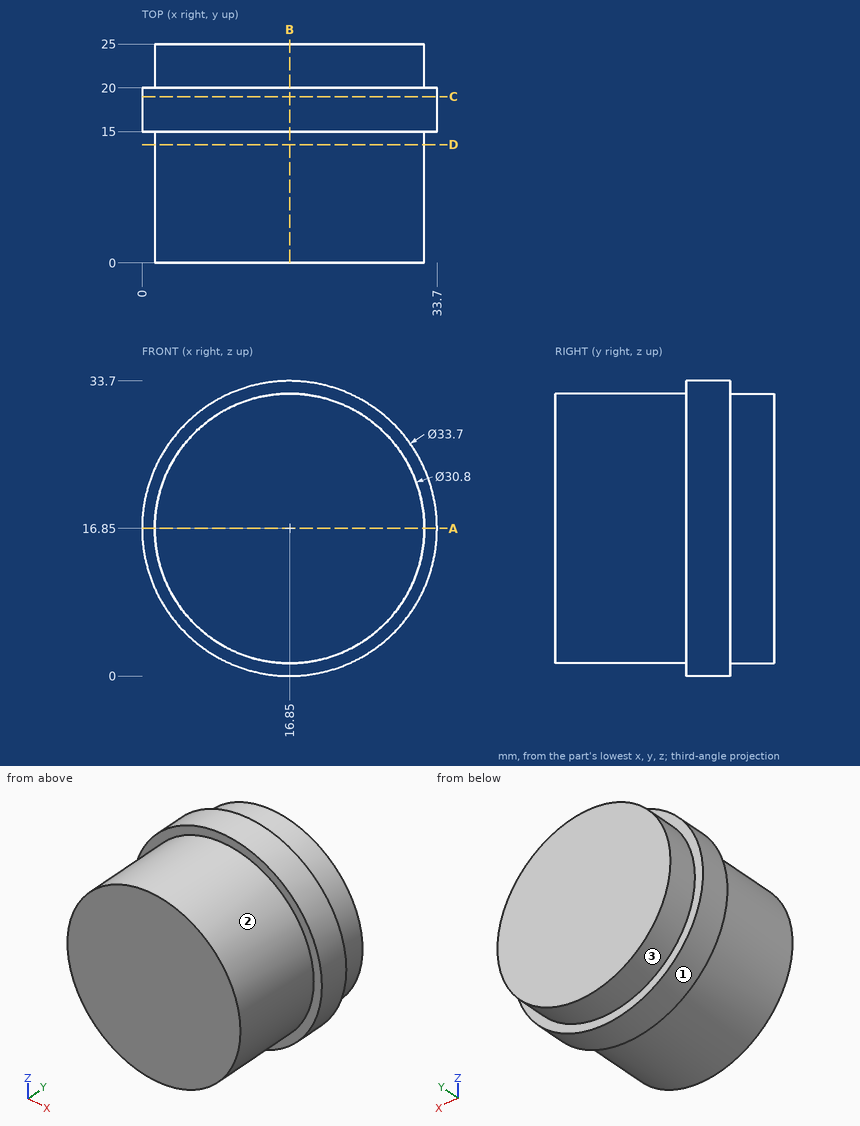
Drawing for the job (mm, zero at the part's lowest x, y, z). A direction names the side the tool comes from. Round coordinates to 2 decimals unless told otherwise and drop trailing zeros. Loops run counter-clockwise (first coordinate to the right, second up) from the corner with the lowest first, then second, coordinate; pieces in that order, holes last. Notation, with made-up numbers: (9.25, -13) - (39.25, -13) arc R12 cw to (39.25, 5) - close; hole circle Ø9 at (40, -9.5). An arc over 180 degrees is marked (long way). Return JSON: item names as keys, results as strings. Group by question number.
Q1. Flat gauge pins, fed straight in: pin 1 Ø1.5 at (y, z) = (14, 3.5) entering from -X; pin 2 Ø12 at (x, y) = (22, 15.5) entering from -Z; pin 3 Ø8 at (y, z) = (7.5, 10.5) entering from -X; pin 4 Ø8 at (y, z) = (16, 7) entering from +X. Where does each tip first touch, or does it go through?
Q2. Band-saw the part on A-A on z = 16.85. Give the cut face in (x, y), plus the area to 4 significant figures.
Q3. Drill centre lines: line 1 along Y through (x, z) = (8, 30); line 2 along Z through (x, y) = (16, 23.5); line 3 along Z through (x, y) = (31.5, 15.5). Where is each one in solid material? Low to high. Write a range as [from, to].
Q4. Band-saw the part on D-D on y = 13.5. Give the cut face in (x, z), plus the area to 3 significant figures.
Q5. Band-saw the part on C-C on y = 19. Give the cut face in (x, z), plus the area to 3 significant figures.
Q6. Band-saw the part on B-B on x = 16.85. Give the cut face in (y, z).
Q7. Tool access for the marked faces 1, 2 and 3: list every direction of +Z, -Z, +X, -X, +Y, -Y with a clear straight run to the whole face (end or side of a thin tool).
Solutions:
{
 "1": {"pin 1": "stops at x = 8", "pin 2": "stops at z = 0", "pin 3": "stops at x = 1.63", "pin 4": "stops at x = 32.65"},
 "2": {"outline": "(0, 15) - (1.45, 15) - (1.45, 0) - (32.25, 0) - (32.25, 15) - (33.7, 15) - (33.7, 20) - (32.25, 20) - (32.25, 25) - (1.45, 25) - (1.45, 20) - (0, 20) - close", "area": "784.5 mm^2"},
 "3": {"line 1": "y = [15, 20]", "line 2": "z = [1.47, 32.23]", "line 3": "z = [8.53, 25.17]"},
 "4": {"outline": "circle Ø30.8 at (16.85, 16.85)", "area": "745 mm^2"},
 "5": {"outline": "circle Ø33.7 at (16.85, 16.85)", "area": "892 mm^2"},
 "6": {"outline": "(0, 1.45) - (15, 1.45) - (15, 0) - (20, 0) - (20, 1.45) - (25, 1.45) - (25, 32.25) - (20, 32.25) - (20, 33.7) - (15, 33.7) - (15, 32.25) - (0, 32.25) - close"},
 "7": {"face 1": "+Y, -Y", "face 2": "-Y", "face 3": "+Y"}
}
